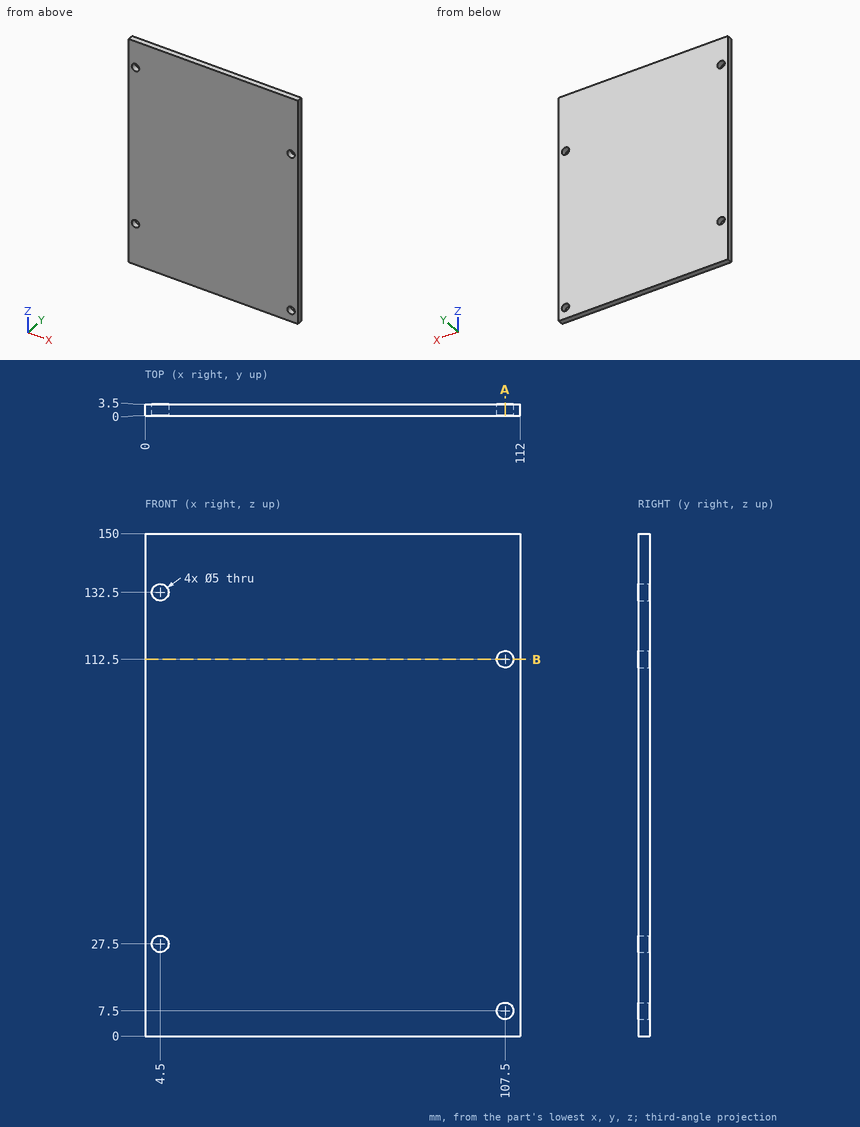
Drawing for the job (mm, zero at the part's lowest x, y, z). Round coordinates to 2 decimals unless told otherwise and drop trailing zeros. Write each loop counter-clockwise with the first axis right and the second up, starting at its lowest first coordinate (ties: lowest second). Pieces come first, ordered by that corner, then holes. Notation, with made-up numbers: (-24, 14) - (21, 14) arc R16 ccw to (21, 21) - close; hole circle Ø4 at (-4, 26.25). An arc over 180 degrees is marked (long way). Use CSV: the item, a comma, the result in double quotes.
(1) Wall check: line 1 (Z direction, x = 107.5, y = 1.2); line 2 (Z direction, x = 4.5, y = 2.1); line 3 (X direction, y = 0.5, z = 113). Give the ranges that are in metal, low to high.
Response:
line 1,"0 to 5, 10 to 110, 115 to 150"
line 2,"0 to 25, 30 to 130, 135 to 150"
line 3,"0 to 105.05, 109.95 to 112"
(2) Pin check, flat tip, straight feed: P1, Ø6, axis at x = 4.5, z = 27.5, coming from the +Y side. Stop position of the tip, or through.
Response:
P1,"y = 3.5"
(3) Band-saw the part on A-A (x = 107.5). Write the cut outline in (y, z), plus the area to 3 significant figures.
Response:
outline,"(0, 0) - (3.5, 0) - (3.5, 5) - (0, 5) - close; (0, 10) - (3.5, 10) - (3.5, 110) - (0, 110) - close; (0, 115) - (3.5, 115) - (3.5, 150) - (0, 150) - close"
area,"490 mm²"
(4) Band-saw the part on B-B (z = 112.5). Write the cut outline in (x, y).
Response:
outline,"(0, 0) - (105, 0) - (105, 3.5) - (0, 3.5) - close; (110, 0) - (112, 0) - (112, 3.5) - (110, 3.5) - close"
